Can you work these out from the drawing? Everything is in mm from the part's minimum corner. Round coordinates to 2 decimals unless told otherwise and drop trailing zeros. Loops run counter-clockwise (first coordinate to the right, second up) from the corner with the lowest first, then second, coordinate; pieces in that order, holes last. Notation, with made-up numbers: (65.25, 35) -> (83.25, 35) arc R26 ccw to (83.25, 61) -> close; hole circle Ø4 at (52.5, 3). An arc over 180 degrees is marked (long way). One line per item, written item: value.
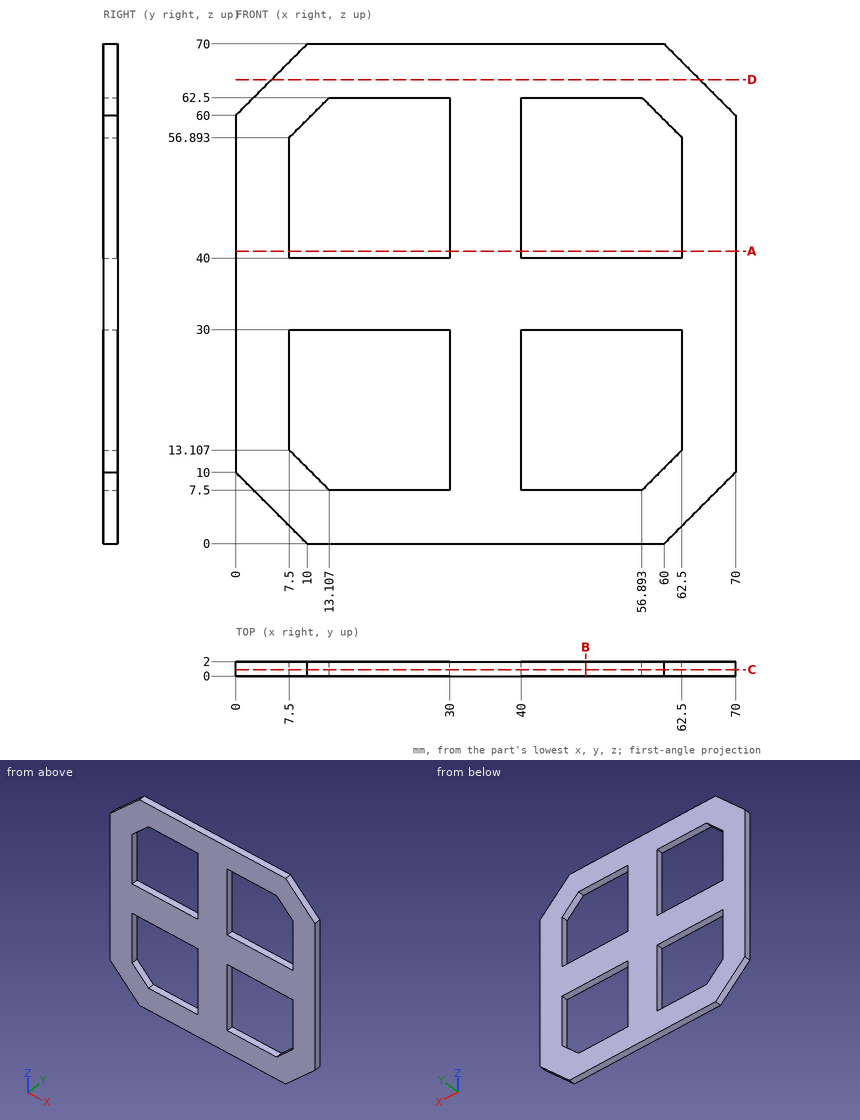
Item 1: If we section it at D-D on z = 65: List the corners of the cut face in (x, y) for me.
Output:
outline: (5, 0) -> (65, 0) -> (65, 2) -> (5, 2) -> close
Item 2: I need wall thicknesses on line 1 (X direction, y = 1.3, z = 43); line 2 (X direction, y = 1.25, z = 59.5) (1 decimal). Which ranges of each line are inside material? Lowest first, please. Write a range as from..to.
Output:
line 1: x = 0..7.5, 30..40, 62.5..70
line 2: x = 0..10.1, 30..40, 59.9..70
Item 3: If we section it at A-A on z = 41: List the corners of the cut face in (x, y) for me, plus the area to 3 significant figures.
Output:
outline: (0, 0) -> (7.5, 0) -> (7.5, 2) -> (0, 2) -> close; (30, 0) -> (40, 0) -> (40, 2) -> (30, 2) -> close; (62.5, 0) -> (70, 0) -> (70, 2) -> (62.5, 2) -> close
area: 50.0 mm²
Item 4: If we section it at C-C on y = 0.9: List the corners of the cut face in (x, z) for me.
Output:
outline: (0, 10) -> (10, 0) -> (60, 0) -> (70, 10) -> (70, 60) -> (60, 70) -> (10, 70) -> (0, 60) -> close; hole (7.5, 13.11) -> (13.11, 7.5) -> (30, 7.5) -> (30, 30) -> (7.5, 30) -> close; hole (7.5, 40) -> (30, 40) -> (30, 62.5) -> (13.11, 62.5) -> (7.5, 56.89) -> close; hole (40, 7.5) -> (56.89, 7.5) -> (62.5, 13.11) -> (62.5, 30) -> (40, 30) -> close; hole (40, 40) -> (62.5, 40) -> (62.5, 56.89) -> (56.89, 62.5) -> (40, 62.5) -> close
Item 5: If we section it at B-B on x = 49: List the corners of the cut face in (y, z) for me.
Output:
outline: (0, 0) -> (2, 0) -> (2, 7.5) -> (0, 7.5) -> close; (0, 30) -> (2, 30) -> (2, 40) -> (0, 40) -> close; (0, 62.5) -> (2, 62.5) -> (2, 70) -> (0, 70) -> close
Item 6: Will this pin go through, and if not, where does the flat tip stop? pin 1 Ø5 at (x, z) = (26.5, 11.5) entering from -Y.
Output:
pin 1: passes through
